Input: part model. Units: mm. Frame: model coordinates. Round coordinates to 2 decimals unless told otherwise and drop trailing zeros. Order: outer loops, then holes, each group sorted by start corner. A loop starts at its lowest first (then second) coordinate and runs counter-clockwise, first axis right, second up. Notation, with made-up numbers: (15.25, 25) - (63.25, 25) arc R15 ccw to (63.25, 33) - close; hole circle Ø3 at (62, 72). An arc over 180 degrees is marked (long way). One line per item, written item: value. Start each with the question number.
from build123d import *

# Parameters (mm, degrees)
BOSS_EXTRUDE1_DEPTH     = 6.35
SKETCH2_R               = 3.3655
CUT_EXTRUDE1_DEPTH      = 7.35
FILLET1_R               = 6.35
CUT_EXTRUDE6_DEPTH      = 7.35
SKETCH4_R               = 3.3655
CUT_EXTRUDE3_DEPTH      = 7.35
CUT_EXTRUDE7_DEPTH      = 7.35
CUT_EXTRUDE8_DEPTH      = 1
CUT_EXTRUDE8_DEPTH_BACK = 7.35


with BuildPart() as part:
    # Sketch1 → Boss-Extrude1 (new body)
    with BuildSketch(Plane(origin=(0, 0, 0), x_dir=(0, 0, -1), z_dir=(1, 0, 0))):
        with BuildLine():
            Line((0, 0), (0, -609.6))
            Line((0, -609.6), (50.8, -609.6))
            ThreePointArc((50.8, -609.6), (194.484097937, -550.084097937), (254, -406.4))
            Line((254, -406.4), (254, 0))
            Line((254, 0), (0, 0))
        make_face()
    extrude(amount=BOSS_EXTRUDE1_DEPTH)

    # Sketch2 → Cut-Extrude1 (cut, through all)
    with BuildSketch(Plane(origin=(6.35, 0, 0), x_dir=(0, 0, -1), z_dir=(1, 0, 0))):
        with Locations((241.3, -25.4)):
            Circle(SKETCH2_R)
        with Locations((12.7, -596.9)):
            Circle(SKETCH2_R)
        with Locations((185.503841816, -541.103841816)):
            Circle(SKETCH2_R)
        with Locations((19.05, -25.4)):
            Circle(SKETCH2_R)
    extrude(amount=-CUT_EXTRUDE1_DEPTH, mode=Mode.SUBTRACT)

    # Fillet1
    fillet1_edges = [part.edges().sort_by_distance(p)[0] for p in [
        (3.175, 0, -254),
        (3.175, -609.6, 0),
        (3.175, 0, 0),
    ]]
    fillet(fillet1_edges, radius=FILLET1_R)

    # Sketch3 → Cut-Extrude6 (cut, through all)
    with BuildSketch(Plane(origin=(6.35, 0, 0), x_dir=(0, 0, -1), z_dir=(1, 0, 0))):
        with BuildLine():
            Line((50.8, -7.62), (101.6, -7.62))
            ThreePointArc((101.6, -7.62), (103.505, -9.525), (101.6, -11.43))
            Line((101.6, -11.43), (50.8, -11.43))
            ThreePointArc((50.8, -11.43), (48.895, -9.525), (50.8, -7.62))
        make_face()
        with BuildLine():
            Line((152.4, -7.62), (203.2, -7.62))
            ThreePointArc((203.2, -7.62), (205.105, -9.525), (203.2, -11.43))
            Line((203.2, -11.43), (152.4, -11.43))
            ThreePointArc((152.4, -11.43), (150.495, -9.525), (152.4, -7.62))
        make_face()
    extrude(amount=-CUT_EXTRUDE6_DEPTH, mode=Mode.SUBTRACT)

    # Sketch4 → Cut-Extrude3 (cut, through all)
    with BuildSketch(Plane(origin=(6.35, 0, 0), x_dir=(0, 0, -1), z_dir=(1, 0, 0))):
        with Locations((9.525, -38.1)):
            Circle(SKETCH4_R)
        with Locations((9.525, -406.4)):
            Circle(SKETCH4_R)
        with Locations((9.525, -571.5)):
            Circle(SKETCH4_R)
    extrude(amount=-CUT_EXTRUDE3_DEPTH, mode=Mode.SUBTRACT)

    # Sketch6 → Cut-Extrude7 (cut, through all)
    with BuildSketch(Plane(origin=(6.35, 0, 0), x_dir=(0, 0, -1), z_dir=(1, 0, 0))):
        with BuildLine():
            Line((234.95, -65.0875), (234.95, -169.8625))
            ThreePointArc((234.95, -169.8625), (233.045, -171.7675), (231.14, -169.8625))
            Line((231.14, -169.8625), (231.14, -65.0875))
            ThreePointArc((231.14, -65.0875), (233.045, -63.1825), (234.95, -65.0875))
        make_face()
        with BuildLine():
            Line((231.14, -379.4125), (231.14, -274.6375))
            ThreePointArc((231.14, -274.6375), (233.045, -272.7325), (234.95, -274.6375))
            Line((234.95, -274.6375), (234.95, -379.4125))
            ThreePointArc((234.95, -379.4125), (233.045, -381.3175), (231.14, -379.4125))
        make_face()
    extrude(amount=-CUT_EXTRUDE7_DEPTH, mode=Mode.SUBTRACT)

    # Sketch7 → Cut-Extrude8 (cut, two sides)
    with BuildSketch(Plane(origin=(6.35, 0, 0), x_dir=(0, 0, -1), z_dir=(1, 0, 0))) as cut_extrude8_sk:
        with BuildLine():
            Line((9.525, -586.74), (41.275, -586.74))
            ThreePointArc((41.275, -586.74), (43.18, -588.645), (41.275, -590.55))
            Line((41.275, -590.55), (9.525, -590.55))
            ThreePointArc((9.525, -590.55), (7.62, -588.645), (9.525, -586.74))
        make_face()
    extrude(amount=CUT_EXTRUDE8_DEPTH, mode=Mode.SUBTRACT)
    extrude(cut_extrude8_sk.sketch, amount=-CUT_EXTRUDE8_DEPTH_BACK, mode=Mode.SUBTRACT)


solid = part.part
Item 1: Section query C-C on z = -120.5. Return loops of the section in (x, y).
Item 2: Line query: L1, parallel to Y at x = 3, z = -19.05; L2, parallel to Y at x = 4, z = -21; L3, parallel to Z at x = 3.25, y = -285. Output: solid intervals per line, ascending.
Item 3: Section query A-A on y = -158. Return loops of the section in (x, z), and give its area (3 significant figures).
Item 4: Section query B-B on x = 1.5. Give the number of separate pieces and of enclosed holes in the cut face, and give its area (3 significant figures).
Geometry results:
1. outline: (0, -597.27) - (6.35, -597.27) - (6.35, 0) - (0, 0) - close
2. L1: y = -609.6 to -590.55, -586.74 to -28.77, -22.03 to 0
2. L2: y = -609.6 to -590.55, -586.74 to -28.14, -22.66 to 0
2. L3: z = -254 to -234.95, -231.14 to 0
3. outline: (0, -254) - (6.35, -254) - (6.35, -234.95) - (0, -234.95) - close; (0, -231.14) - (6.35, -231.14) - (6.35, 0) - (0, 0) - close
3. area: 1,590 mm^2
4. separate pieces: 1
4. enclosed holes: 12
4. area: 144,000 mm^2
